The figure shows three views and two pictorial views of one solid part (mm, origin at its lowest corner). Answer the questions. A direction names the side the tool comes from. Coordinates: 2 decimals unless noted, no trailing zeros. Loops run counter-clockwise (first coordinate to the right, second up) from the corner with the lowest first, then second, coordinate; pieces in that order, holes last. Notation, with made-up numbers: M 3.25,-8.5 L 20.25,-8.5 A8 ccw 20.25,-4.5 Z; hole C -28.5,-14 d3. An arc over 180 degrees is marked long. Return JSON: item names as keys, results as strings. Group by question number.
1. Given P1, Ø1.5, axis at x = 30.5, y = 6.5, coming from the -Z side; P2, Ø5, axis at x = 17.6, y = 30.1, coming from the +Z side; P3, Ø17.5, axis at x = 21.5, y = 13, coming from the +Z side; P4, Ø5, axis at y = 6, z = 9, coming from the +X side, each flat-ended and moving along its own axis, determine where each tip first touches the part or whether it passes through.
2. Which of the six approach directions +Z, -Z, +X, -X, +Y, -Y give full straight-line access (tool end or side, diameter ignored) to the marked faces 1 and 2?
3. Section D-D (z = 48) is taken. Write down the section's boundary in (x, y), then the cut area to 3 significant figures.
4. Section A-A (z = 4) is taken. Write down the section's boundary in (x, y), then the cut area to 3 significant figures.
5. Straight lines are drawn through the part: L1, parallel to Y at x = 17.6, z = 2.7; L2, parallel to X at y = 17, z = 3; L3, parallel to Z at x = 30.5, y = 9. For each, find the intervals that lie inside material, in ascending order. Write a range as from..to.
6. Section C-C (x = 8.1) is taken. Write down the section's boundary in (y, z), then the cut area to 3 significant figures.
7. Section B-B (y = 17.6) is taken. Write down the section's boundary in (x, z).
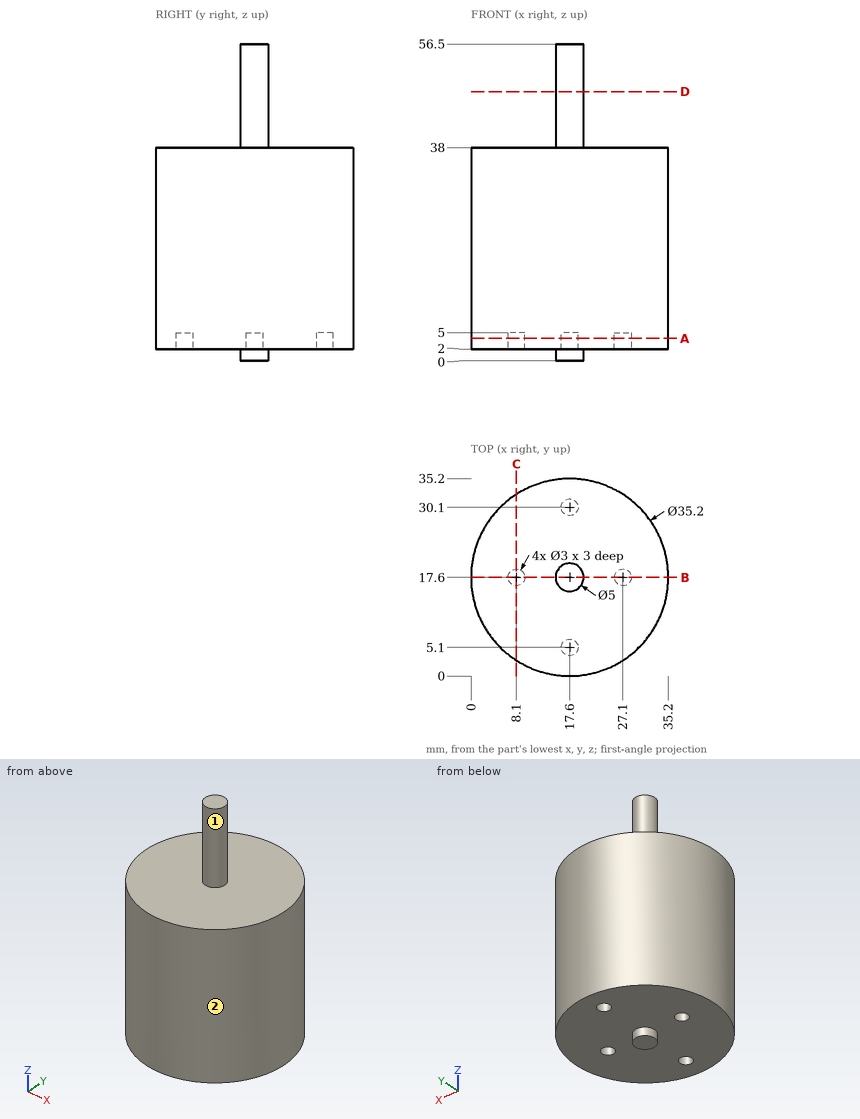
Worked out:
{
 "1": {"P1": "z = 2", "P2": "z = 38", "P3": "z = 56.5", "P4": "x = 32.66"},
 "2": {"face 1": "+Z", "face 2": "+Z, -Z"},
 "3": {"outline": "C 17.6,17.6 d5", "area": "19.6 mm^2"},
 "4": {"outline": "C 17.6,17.6 d35.2; hole C 8.1,17.6 d3; hole C 17.6,5.1 d3; hole C 17.6,30.1 d3; hole C 27.1,17.6 d3", "area": "945 mm^2"},
 "5": {"L1": "0..3.6, 6.6..28.6, 31.6..35.2", "L2": "0.01..6.73, 9.47..25.73, 28.47..35.19", "L3": "2..38"},
 "6": {"outline": "M 2.78,2 L 16.1,2 L 16.1,5 L 19.1,5 L 19.1,2 L 32.42,2 L 32.42,38 L 2.78,38 Z", "area": "1,060 mm^2"},
 "7": {"outline": "M 0,2 L 6.6,2 L 6.6,5 L 9.6,5 L 9.6,2 L 15.1,2 L 15.1,0 L 20.1,0 L 20.1,2 L 25.6,2 L 25.6,5 L 28.6,5 L 28.6,2 L 35.2,2 L 35.2,38 L 20.1,38 L 20.1,56.5 L 15.1,56.5 L 15.1,38 L 0,38 Z"}
}
